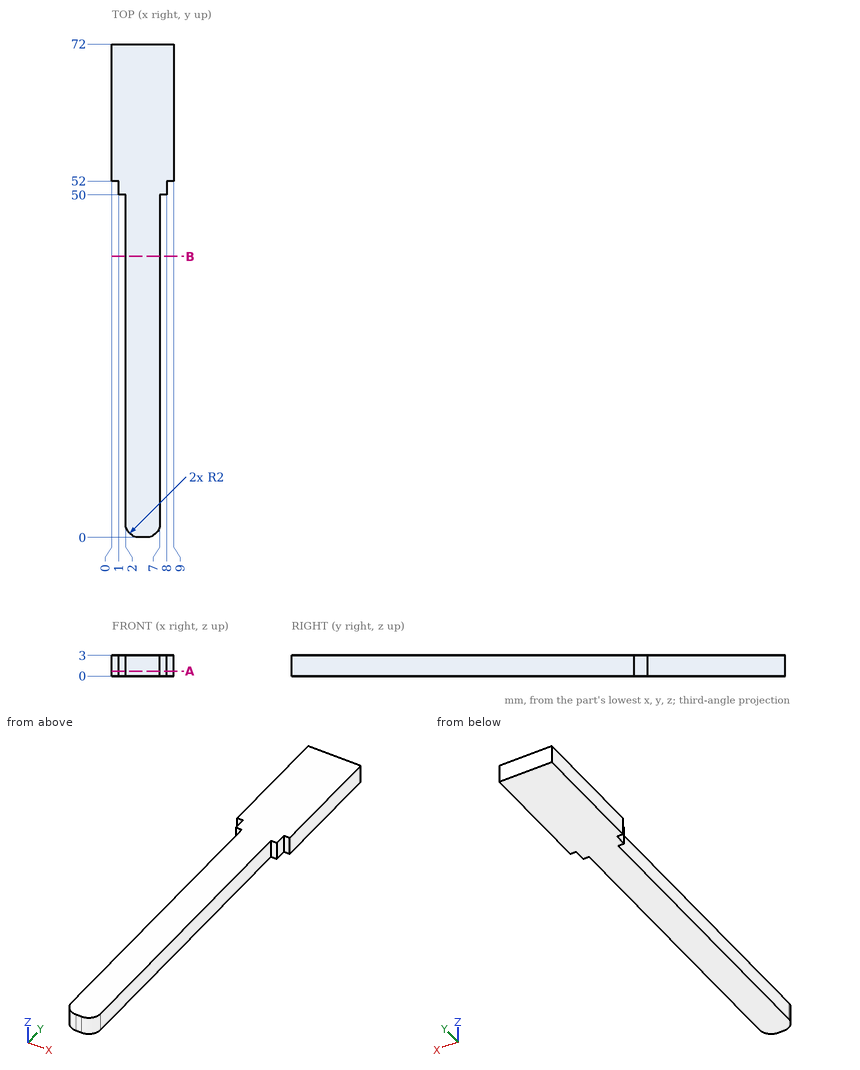
Check sheet for the drawn part. Datum: minimum x, y, z corner. Units: mm. Coordinates: 2 decimals unless noted, no trailing zeros. Order: outer loops, then holes, each group sorted by start corner. A loop starts at its lowest first (then second) coordinate and runs counter-clockwise, first axis right, second up. Notation, with made-up numbers: M -32.5,-1.75 L 0.5,-1.75 A21 cw 0.5,26.25 Z; hole C -4,41 d11. An arc over 180 degrees is marked long. One line per question, with ' | ' between items. Start each with the question number.
Item 1: Gauge pin test, flat ends, axial feed: pin 1 (0.9 mm diameter, centred on y = 25, z = 1, fed in from -X); pin 2 (1.5 mm diameter, centred on y = 33.5, z = 1.5, fed in from +X); pin 3 (0.6 mm diameter, centred on y = 51, z = 1, fed in from -X). Record the tip position at first contact, or that the pin passes through.
Item 2: Cross-section at B-B on y = 41. Enter the section's corners in (x, z), then the cut area to 3 significant figures.
Item 3: Cross-section at A-A on z = 0.7. Enter the section's corners in (x, y), then the cut area to 3 significant figures.
Item 4: Material ranges on L1, parallel to X at y = 26, z = 1.1; L2, parallel to Y at x = 1.25, z = 0.35; L3, parallel to X at y = 51, z = 0.4, recorded low to high. Write a range as [from, to].
Findings:
1) pin 1: stops at x = 2 | pin 2: stops at x = 7 | pin 3: stops at x = 1
2) outline: M 2,0 L 7,0 L 7,3 L 2,3 Z | area: 15.0 mm²
3) outline: M 0,52 L 1,52 L 1,50 L 2,50 L 2,2 A2 ccw 4,0 L 5,0 A2 ccw 7,2 L 7,50 L 8,50 L 8,52 L 9,52 L 9,72 L 0,72 Z | area: 442 mm²
4) L1: x = [2, 7] | L2: y = [50, 72] | L3: x = [1, 8]
